Model file for the job. Use its own axes, mm. Face numbers are marked on the shaded views. A direction names the side the tool comes from. Give positions to 0.01 mm unless a question says otherwise; leave off trailing zeros. Order: outer loops, then holes, each group sorted by start corner. A loop starts at its lowest first (then second) coordinate and runs counter-clockwise, first axis right, second up. Notation, with made-up numbers: (50, 2) -> (56, 2) arc R17 ccw to (56, 17) -> close; hole circle Ø2 at (-18.5, 31). An arc over 180 degrees is marked (long way). Answer in a Markdown table with one row per item. Add a question column.
from build123d import *

# Parameters (mm, degrees)
SKIZZE1_W                                    = 106
SKIZZE1_H                                    = 120
AUFSATZ_LINEAR_AUSTRAGEN1_DEPTH              = 36
WANDUNG1_T                                   = -2
SKIZZE2_R                                    = 4.5
AUFSATZ_LINEAR_AUSTRAGEN2_DEPTH              = 4
VERRUNDUNG1_R                                = 2
STIRNSENKUNG_F_R_M3_ZYLINDERSCHRAUBE_2_COUNT = 2
STIRNSENKUNG_F_R_M3_ZYLINDERSCHRAUBE_2_PITCH = 140.889047126
STIRNSENKUNG_F_R_M3_ZYLINDERSCHRAUBE_3_COUNT = 2
STIRNSENKUNG_F_R_M3_ZYLINDERSCHRAUBE_3_PITCH = 105
STIRNSENKUNG_F_R_M3_ZYLINDERSCHRAUBE_4_COUNT = 2
STIRNSENKUNG_F_R_M3_ZYLINDERSCHRAUBE_4_PITCH = 93.94
SKIZZE7_W                                    = 17
SKIZZE7_H                                    = 14.6
SCHNITT_LINEAR_AUSTRAGEN1_DEPTH              = 10
SKIZZE8_W                                    = 8.16
SKIZZE8_H                                    = 13.4
SCHNITT_LINEAR_AUSTRAGEN2_DEPTH              = 10
LINEARES_MUSTER2_COUNT                       = 2
LINEARES_MUSTER2_PITCH                       = 27.85
LINEARES_MUSTER3_COUNT                       = 2
LINEARES_MUSTER3_PITCH                       = 53.76
LINEARES_MUSTER4_COUNT                       = 2
LINEARES_MUSTER4_PITCH                       = 81.35
SKIZZE10_W                                   = 5
SKIZZE10_H                                   = 3
SCHNITT_LINEAR_AUSTRAGEN3_DEPTH              = 3


with BuildPart() as part:
    # Skizze1 → Aufsatz-Linear austragen1 (new body)
    with BuildSketch(Plane(origin=(0, 0, 0), x_dir=(1, 0, 0), z_dir=(0, 1, 0))):
        with Locations((53, 60)):
            Rectangle(SKIZZE1_W, SKIZZE1_H)
    extrude(amount=AUFSATZ_LINEAR_AUSTRAGEN1_DEPTH)

    # Wandung1
    wandung1_openings = [part.faces().sort_by_distance(p)[0] for p in [
        (53, 36, -60),
    ]]
    offset(amount=WANDUNG1_T, openings=wandung1_openings, kind=Kind.INTERSECTION)

    # Skizze2 → Aufsatz-Linear austragen2 (add)
    with BuildSketch(Plane(origin=(0, 2, 0), x_dir=(1, 0, 0), z_dir=(0, 1, 0))):
        with Locations((6, 7.5)):
            Circle(SKIZZE2_R)
        with Locations((99.94, 7.5)):
            Circle(SKIZZE2_R)
        with Locations((99.94, 112.5)):
            Circle(SKIZZE2_R)
        with Locations((6, 112.5)):
            Circle(SKIZZE2_R)
    extrude(amount=AUFSATZ_LINEAR_AUSTRAGEN2_DEPTH)

    # Verrundung1
    verrundung1_edges = [part.edges().sort_by_distance(p)[0] for p in [
        (0, 18, -120),
        (106, 18, -120),
        (106, 18, 0),
        (0, 18, 0),
    ]]
    fillet(verrundung1_edges, radius=VERRUNDUNG1_R)

    # Skizze6 → Stirnsenkung für M3 Zylinderschraube mit Innensechskant1 (revolve, cut)
    with BuildSketch(Plane(origin=(100, 0, -7.5), x_dir=(0, 0, -1), z_dir=(1, 0, 0))):
        Polygon((0, 0), (0, 15.021463052), (1.7, 14), (1.7, 3.4), (3.25, 3.4), (3.25, 0.025), (3.275, 0), align=None)
    stirnsenkung_f_r_m3_zylinderschraube_mit = revolve(axis=Axis((100, -6.35, -7.5), (0, 1, 0)), mode=Mode.SUBTRACT)

    # Stirnsenkung f_r M3 Zylinderschraube 2: Stirnsenkung für M3 Zylinderschraube mit Innensechskant1 ×2
    with Locations(*[Vector(-0.6667658126480086, 0, -0.7452673017675208) * (i * STIRNSENKUNG_F_R_M3_ZYLINDERSCHRAUBE_2_PITCH) for i in range(1, STIRNSENKUNG_F_R_M3_ZYLINDERSCHRAUBE_2_COUNT)]):
        add(stirnsenkung_f_r_m3_zylinderschraube_mit, mode=Mode.SUBTRACT)

    # Stirnsenkung f_r M3 Zylinderschraube 3: Stirnsenkung für M3 Zylinderschraube mit Innensechskant1 ×2
    with Locations(*[(0, 0, -i * STIRNSENKUNG_F_R_M3_ZYLINDERSCHRAUBE_3_PITCH) for i in range(1, STIRNSENKUNG_F_R_M3_ZYLINDERSCHRAUBE_3_COUNT)]):
        add(stirnsenkung_f_r_m3_zylinderschraube_mit, mode=Mode.SUBTRACT)

    # Stirnsenkung f_r M3 Zylinderschraube 4: Stirnsenkung für M3 Zylinderschraube mit Innensechskant1 ×2
    with Locations(*[(-i * STIRNSENKUNG_F_R_M3_ZYLINDERSCHRAUBE_4_PITCH, 0, 0) for i in range(1, STIRNSENKUNG_F_R_M3_ZYLINDERSCHRAUBE_4_COUNT)]):
        add(stirnsenkung_f_r_m3_zylinderschraube_mit, mode=Mode.SUBTRACT)

    # Skizze7 → Schnitt-Linear austragen1 (cut)
    with BuildSketch(Plane.ZY):
        with Locations((-21.75, 14.72)):
            Rectangle(SKIZZE7_W, SKIZZE7_H)
    extrude(amount=-SCHNITT_LINEAR_AUSTRAGEN1_DEPTH, mode=Mode.SUBTRACT)

    # Skizze8 → Schnitt-Linear austragen2 (cut)
    with BuildSketch(Plane(origin=(106, 0, 0), x_dir=(0, 0, -1), z_dir=(1, 0, 0))):
        with Locations((14.06, 17.42)):
            Rectangle(SKIZZE8_W, SKIZZE8_H)
        with Locations((24.22, 17.42)):
            Rectangle(SKIZZE8_W, SKIZZE8_H)
    schnitt_linear_austragen2 = extrude(amount=-SCHNITT_LINEAR_AUSTRAGEN2_DEPTH, mode=Mode.SUBTRACT)

    # Lineares Muster2: Schnitt-Linear austragen2 ×2
    with Locations(*[(0, 0, -i * LINEARES_MUSTER2_PITCH) for i in range(1, LINEARES_MUSTER2_COUNT)]):
        add(schnitt_linear_austragen2, mode=Mode.SUBTRACT)

    # Lineares Muster3: Schnitt-Linear austragen2 ×2
    with Locations(*[(0, 0, -i * LINEARES_MUSTER3_PITCH) for i in range(1, LINEARES_MUSTER3_COUNT)]):
        add(schnitt_linear_austragen2, mode=Mode.SUBTRACT)

    # Lineares Muster4: Schnitt-Linear austragen2 ×2
    with Locations(*[(0, 0, -i * LINEARES_MUSTER4_PITCH) for i in range(1, LINEARES_MUSTER4_COUNT)]):
        add(schnitt_linear_austragen2, mode=Mode.SUBTRACT)

    # Skizze10 → Schnitt-Linear austragen3 (cut)
    with BuildSketch(Plane.ZY):
        with Locations((-21.75, 5.92)):
            Rectangle(SKIZZE10_W, SKIZZE10_H)
    extrude(amount=-SCHNITT_LINEAR_AUSTRAGEN3_DEPTH, mode=Mode.SUBTRACT)


solid = part.part
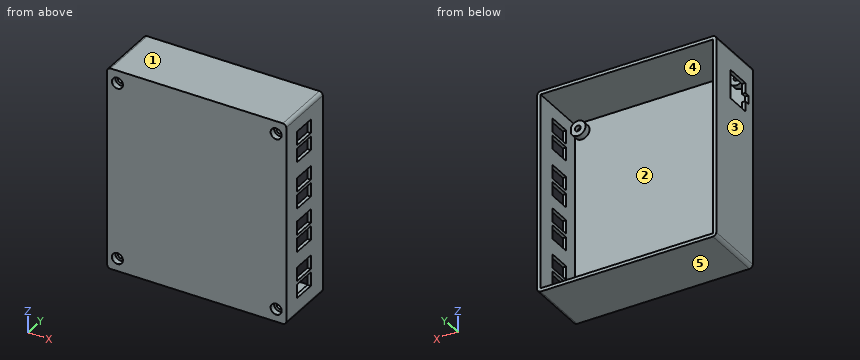
Item 1: Which spindle directions (+Z, -Z, +X, -X, +Y, -Y) get a long thin tool onto all of the face, cutting with end or side? Do the marked faces 4 and 5. Say none if no direction does.
Item 2: Saw through at B-B on z = -75.5. List the corners of the cut face in (x, y).
Item 3: Saw through at A-A on z = -112.5. Give the number of separate pieces and of enclosed holes in the cut face, plus the area to 3 significant figures.
Item 4: Two-plate mould, pull along X, no slides. Class the marked faces 1, 2 and 3: pulls with the +X half, pulls with the -X half, needs draft (parallel to the pull), parting line crosses it, or undercut.
Item 5: Saw through at D-D on x = 50. List the corners of the cut face in (y, z).
Item 6: Wall check: line 1 (X direction, y = 5, z = -7.5); line 2 (Z direction, x = 100, y = 5); line 3 (X direction, y = 21.5, z = -82.5). Give the ranges that are in metal, low to high.
Item 7: Pin check, flat tips, straight feed: pin 1 Ø1.6 at (x, y) = (1.5, 6) entering from -Z; pin 2 Ø1.6 at (x, y) = (105.5, 16.5) entering from -Z; pin 3 Ø1.6 at (x, y) = (105, 18.5) entering from +Z; pin 4 Ø0.6 at (x, y) = (1, 5.5) entering from +Z. Stop position of each tip, or through.
Evaluation:
| question | item | result |
|---|---|---|
| 1 | face 4 | +Y |
| 1 | face 5 | -Z, +X, -X, +Y, -Y |
| 2 | outline | (0, 0) -> (106, 0) -> (106, 10.72) -> (104, 10.72) -> (104, 2) -> (2, 2) -> (2, 36) -> (0, 36) -> close; (104, 24.12) -> (106, 24.12) -> (106, 36) -> (104, 36) -> close |
| 3 | separate pieces | 3 |
| 3 | enclosed holes | 0 |
| 3 | area | 354 mm2 |
| 4 | face 1 | needs draft |
| 4 | face 2 | undercut |
| 4 | face 3 | pulls with the -X half |
| 5 | outline | (0, -120) -> (36, -120) -> (36, -118) -> (2, -118) -> (2, -2) -> (36, -2) -> (36, 0) -> (0, 0) -> close |
| 6 | line 1 | x = 0 to 4.36, 7.76 to 10.5, 95.44 to 98.3, 101.7 to 106 |
| 6 | line 2 | z = -120 to -118, -117 to -114.2, -110.8 to -108, -12 to -9.2, -5.8 to -3, -2 to 0 |
| 6 | line 3 | x = 0 to 2, 104 to 106 |
| 7 | pin 1 | stops at z = -120 |
| 7 | pin 2 | stops at z = -119.87 |
| 7 | pin 3 | stops at z = -0.01 |
| 7 | pin 4 | stops at z = -0.13 |
